Read the model definition and answer for the solid it produces. Units are mm, in the model's axes. A direction names the side the tool comes from. Give positions to 0.01 mm unless a question says otherwise; leave off trailing zeros. Write each loop counter-clockwise with the first axis right and the second up, starting at its lowest first coordinate (ties: lowest second). Pieces come first, ordered by that corner, then holes.
```python
from build123d import *

# Parameters (mm, degrees)
SKETCH2_R                = 13
BOSS_EXTRUDE1_DEPTH      = 12.7
M5_CLEARANCE_HOLE1_D     = 5.5
M5_CLEARANCE_HOLE1_DEPTH = 10.1
M5_CLEARANCE_HOLE1_TIP   = 1.652366702
BOSS_EXTRUDE2_DEPTH      = 3.5
SKETCH10_R               = 13
CUT_EXTRUDE1_DEPTH       = 1.7
SKETCH11_R               = 7.5
CUT_EXTRUDE2_DEPTH       = 17.2
M3_CLEARANCE_HOLE1_D     = 3.4
M3_CLEARANCE_HOLE1_DEPTH = 7.5
M3_CLEARANCE_HOLE1_TIP   = 1.021463052


with BuildPart() as part:
    # Sketch2 → Boss-Extrude1 (new body)
    with BuildSketch(Plane(origin=(0, 0, 0), x_dir=(1, 0, 0), z_dir=(0, 1, 0))):
        with BuildLine():
            Line((-30, 9), (-17.5, 9))
            Line((-17.5, 9), (-17.5, 0))
            ThreePointArc((-17.5, 0), (0, -17.5), (17.5, 0))
            Line((17.5, 0), (17.5, 9))
            Line((17.5, 9), (30, 9))
            Line((30, 9), (30, 19))
            Line((30, 19), (-30, 19))
            Line((-30, 19), (-30, 9))
        make_face()
        Circle(SKETCH2_R, mode=Mode.SUBTRACT)
    extrude(amount=BOSS_EXTRUDE1_DEPTH)

    # M5 Clearance Hole1
    with Locations(Plane(origin=(-25, 6.35, -19), x_dir=(-1, 0, 0), z_dir=(0, 0, -1))):
        with Locations((0, 0), (-50, 0)):
            Hole(M5_CLEARANCE_HOLE1_D / 2, depth=M5_CLEARANCE_HOLE1_DEPTH)
            with Locations((0, 0, -(M5_CLEARANCE_HOLE1_DEPTH + M5_CLEARANCE_HOLE1_TIP / 2))):  # 118° drill point
                Cone(0, M5_CLEARANCE_HOLE1_D / 2, M5_CLEARANCE_HOLE1_TIP, mode=Mode.SUBTRACT)

    # Sketch9 → Boss-Extrude2 (add)
    with BuildSketch(Plane(origin=(0, 12.7, 0), x_dir=(1, 0, 0), z_dir=(0, 1, 0))):
        with BuildLine():
            Line((-30, 9), (-17.5, 9))
            Line((-17.5, 9), (-17.5, 0))
            ThreePointArc((-17.5, 0), (0, -17.5), (17.5, 0))
            Line((17.5, 0), (17.5, 9))
            Line((17.5, 9), (30, 9))
            Line((30, 9), (30, 19))
            Line((30, 19), (-30, 19))
            Line((-30, 19), (-30, 9))
        make_face()
    extrude(amount=BOSS_EXTRUDE2_DEPTH)

    # Sketch10 → Cut-Extrude1 (cut)
    with BuildSketch(Plane.XZ.offset(-12.7)):
        Circle(SKETCH10_R)
    extrude(amount=-CUT_EXTRUDE1_DEPTH, mode=Mode.SUBTRACT)

    # Sketch11 → Cut-Extrude2 (cut, through all)
    with BuildSketch(Plane(origin=(0, 16.2, 0), x_dir=(1, 0, 0), z_dir=(0, 1, 0))):
        Circle(SKETCH11_R)
    extrude(amount=-CUT_EXTRUDE2_DEPTH, mode=Mode.SUBTRACT)

    # M3 Clearance Hole1
    with Locations(Plane(origin=(-10, 16.2, 0), x_dir=(0, 0, 1), z_dir=(0, 1, 0))):
        with Locations((0, 0), (10, 10), (0, 20), (-10, 10)):
            Hole(M3_CLEARANCE_HOLE1_D / 2, depth=M3_CLEARANCE_HOLE1_DEPTH)
            with Locations((0, 0, -(M3_CLEARANCE_HOLE1_DEPTH + M3_CLEARANCE_HOLE1_TIP / 2))):  # 118° drill point
                Cone(0, M3_CLEARANCE_HOLE1_D / 2, M3_CLEARANCE_HOLE1_TIP, mode=Mode.SUBTRACT)


solid = part.part
```
Item 1: Each of these flat-tipped pins is pushed along its axis until it touches: pin 1 Ø4.5 at (x, z) = (0, -10) entering from -Y; pin 2 Ø8 at (y, z) = (4, -3) entering from -X; pin 3 Ø1.5 at (x, y) = (-3.5, 8.5) entering from +Z. Where does it stop, or does it pass through?
Result set:
pin 1: stops at y = 14.4
pin 2: stops at x = -17.5
pin 3: stops at z = 17.28
Item 2: Section D-D (y = 11) is taken. Write down the section's boundary in (x, z).
Result set:
outline: (-30, -19) - (30, -19) - (30, -9) - (17.5, -9) - (17.5, 0) arc R17.5 ccw to (-17.5, 0) - (-17.5, -9) - (-30, -9) - close; hole circle Ø26 at (0, 0)
Item 3: Section C-C (z = -4.5) is taken. Write down the section's boundary in (x, y).
Result set:
outline: (-17.5, 0) - (-12.2, 0) - (-12.2, 14.4) - (-6, 14.4) - (-6, 16.2) - (-17.5, 16.2) - close; (6, 14.4) - (12.2, 14.4) - (12.2, 0) - (17.5, 0) - (17.5, 16.2) - (6, 16.2) - close
Item 4: Section B-B (x = 25) is taken. Write down the section's boundary in (y, z), and give its area (3 significant figures).
Result set:
outline: (0, -19) - (3.6, -19) - (3.6, -9) - (0, -9) - close; (9.1, -19) - (16.2, -19) - (16.2, -9) - (9.1, -9) - close
area: 107 mm2
Item 5: Section A-A (y = 6.35) is taken. Write down the section's boundary in (x, z).
Result set:
outline: (-30, -19) - (-27.75, -19) - (-27.75, -9) - (-30, -9) - close; (-22.25, -19) - (22.25, -19) - (22.25, -9) - (17.5, -9) - (17.5, 0) arc R17.5 ccw to (-17.5, 0) - (-17.5, -9) - (-22.25, -9) - close; (27.75, -19) - (30, -19) - (30, -9) - (27.75, -9) - close; hole circle Ø26 at (0, 0)
Item 6: Which of the six approach directions +Z, -Z, +X, -X, +Y, -Y give full straight-line access (tool end or side, diameter ignored) to faces 4 (the flat face through (-17.5, 8, -5)), 5 (the flat face through (17.5, 8, -4)), 6 (the cylindrical face through (-10.316, 7.099, 7.91))?
Result set:
face 4: +Z, -X, +Y, -Y
face 5: +Z, +X, +Y, -Y
face 6: -Y
Item 7: Determine the mould class of faces 1 (the flat face through (30, 8, -14)), 2 (the flat face through (-22, 8, -9)), 3 (the cylindrical face through (-1.66, 15.29, -9.63)) for opening direction X: pulls with the +X half, pulls with the -X half, needs draft (parallel to the pull), parting line crosses it, or undercut.
Result set:
face 1: pulls with the +X half
face 2: needs draft
face 3: undercut
Item 8: Find the intervals of material crossed by line 1 along Y through (x, z) = (25, -11); line 2 along X through (y, z) = (15.85, -10); line 3 along Z through (x, y) = (9.5, 1.25), in increasing order.
Result set:
line 1: y = 0 to 3.6, 9.1 to 16.2
line 2: x = -30 to -1.7, 1.7 to 30
line 3: z = -19 to -8.87, 8.87 to 14.7
